Design review of the part shown in the three views and the two pictorial views. Dimensions are in mm from the part's minimum x, y and z. Coordinates: 2 decimals unless noted, no trailing zeros. Loops run counter-clockwise (first coordinate to the right, second up) from the corner with the lowest first, then second, coordinate; pieces in that order, holes last. Notation, with made-up numbers: (68, 7.5) -> (89, 7.5) arc R23 cw to (89, 18.5) -> close; hole circle Ø6 at (-20, -16.5). An arc over 180 degrees is marked (long way). One line per item, written item: value.
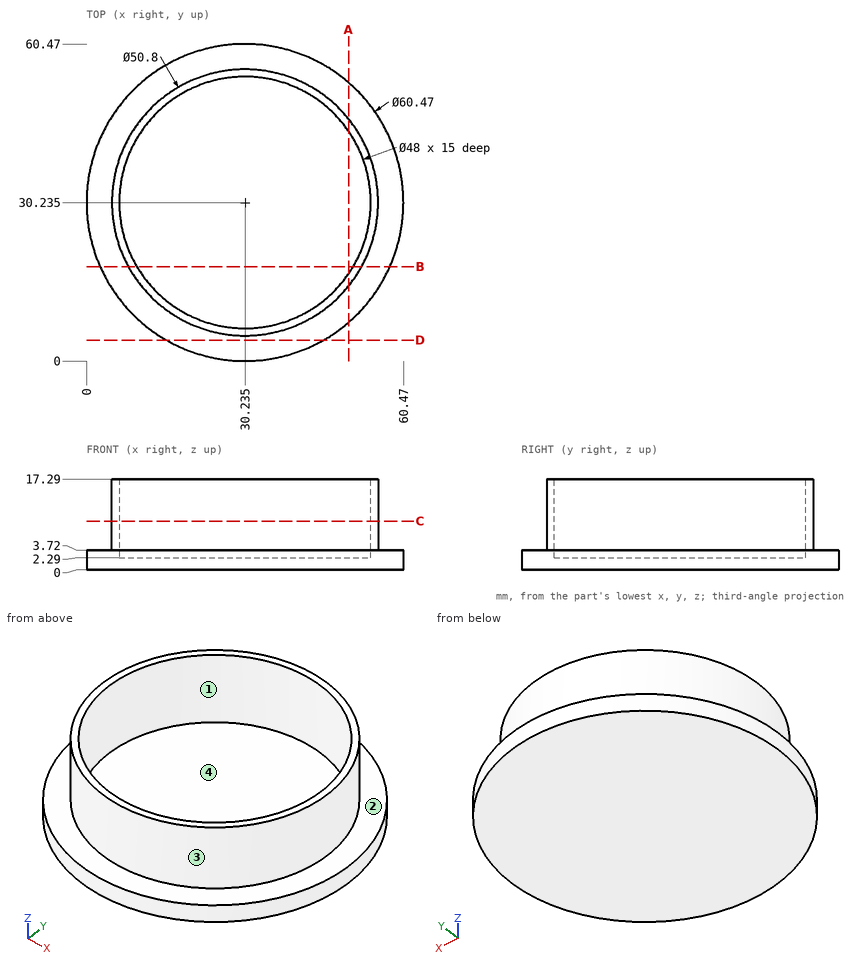
1. Take a section at C-C, the plane z = 9.25. Give the boundary of the cut face in (x, y) (3 decimals), and give its area (3 significant figures).
Return value:
outline: circle Ø50.8 at (30.235, 30.235); hole circle Ø48 at (30.235, 30.235)
area: 217 mm2
2. Take a section at D-D, the plane y = 4. Give the boundary of the cut face in (x, z), and give its area (3 significant figures).
Return value:
outline: (15.21, 0) -> (45.26, 0) -> (45.26, 3.72) -> (15.21, 3.72) -> close
area: 112 mm2
3. Take a section at B-B, the plane y = 18. Give the boundary of the cut face in (x, z).
Return value:
outline: (2.59, 0) -> (57.88, 0) -> (57.88, 3.72) -> (52.49, 3.72) -> (52.49, 17.29) -> (50.88, 17.29) -> (50.88, 2.29) -> (9.59, 2.29) -> (9.59, 17.29) -> (7.98, 17.29) -> (7.98, 3.72) -> (2.59, 3.72) -> close
4. Take a section at A-A, the plane x = 50. Give the boundary of the cut face in (y, z).
Return value:
outline: (7.35, 0) -> (53.12, 0) -> (53.12, 3.72) -> (46.19, 3.72) -> (46.19, 17.29) -> (43.85, 17.29) -> (43.85, 2.29) -> (16.62, 2.29) -> (16.62, 17.29) -> (14.28, 17.29) -> (14.28, 3.72) -> (7.35, 3.72) -> close
5. The part is to be moulded in two halves that separate along X. For the marked faces 1, 2, 3 and 4, say which applies: pulls with the +X half, pulls with the -X half, needs draft (parallel to the pull), parting line crosses it, or undercut.
Return value:
face 1: undercut
face 2: needs draft
face 3: parting line crosses it
face 4: undercut
6. To check wall thickness, follow probe 1 along Z at (x, y) = (40, 37); probe 2 along X at (y, z) = (36.5, 2.5); probe 3 along X at (y, z) = (40, 6.5). State the ranges of each line that lie inside material, in increasing order. Write a range as from..to.
Return value:
probe 1: z = 0..2.29
probe 2: x = 0.66..7.07, 53.4..59.81
probe 3: x = 6.79..8.31, 52.16..53.68
7. Insertion check: pin 1 Ø12 at (x, y) = (11.5, 15.5) entering from +Z; pin 2 Ø6 at (y, z) = (54, 5.5) entering from +X; pin 3 Ø5 at (x, z) = (15, 2) entering from -Y; pin 4 Ø5 at (x, z) = (28.5, 6) entering from +Y. Each pin has a flat end and moves straight along its axis. Give the tip position at first contact, or say it passes through.
Return value:
pin 1: stops at z = 17.29
pin 2: stops at x = 51.64
pin 3: stops at y = 2.81
pin 4: stops at y = 60.46
